```python
from build123d import *

# Parameters (mm, degrees)
ESTRUSIONE_ESTRUSIONE1_DEPTH                         = 25
SCHIZZO3_R                                           = 7
ESTRUSIONE_ESTRUSIONE2_DEPTH                         = 14.91
FORO_LAMATO_PER_VITE_M8_A_TESTA_CILINDRI_D           = 9
FORO_LAMATO_PER_VITE_M8_A_TESTA_CILINDRI_DEPTH       = 34.91
FORO_LAMATO_PER_VITE_M8_A_TESTA_CILINDRI_CBORE_D     = 15
FORO_LAMATO_PER_VITE_M8_A_TESTA_CILINDRI_CBORE_DEPTH = 8.6
TAGLIO_ESTRUSIONE3_DEPTH                             = 150
TAGLIO_ESTRUSIONE4_DEPTH                             = 30
TAGLIO_ESTRUSIONE5_START                             = -20
TAGLIO_ESTRUSIONE5_DEPTH                             = 20
TAGLIO_ESTRUSIONE6_DEPTH                             = 180
TAGLIO_ESTRUSIONE7_START                             = -5
TAGLIO_ESTRUSIONE7_DEPTH                             = 5
TAGLIO_ESTRUSIONE8_DEPTH                             = 2


with BuildPart() as part:
    # Schizzo2 → Estrusione-Estrusione1 (new body)
    with BuildSketch(Plane.XY):
        Polygon((0, 0), (-88, 0), (-88, -200), (-48, -200), (-48, -170), (-68, -170), (-68, -20), (0, -20), align=None)
    extrude(amount=ESTRUSIONE_ESTRUSIONE1_DEPTH)

    # Schizzo3 → Estrusione-Estrusione2 (add)
    with BuildSketch(Plane(origin=(0, 0, 0), x_dir=(1, 0, 0), z_dir=(0, 1, 0))):
        with Locations(Location((-41, -12.5, 0), (0, 0, 180))):
            Circle(SCHIZZO3_R)
        with Locations((-9, -12.5)):
            Circle(SCHIZZO3_R)
    extrude(amount=ESTRUSIONE_ESTRUSIONE2_DEPTH)

    # Foro lamato per Vite M8 a testa cilindrica-1
    with Locations(Plane(origin=(0, -20, 0), x_dir=(-1, 0, 0), z_dir=(0, -1, 0))):
        with Locations((9, -12.5), (41, -12.5)):
            CounterBoreHole(FORO_LAMATO_PER_VITE_M8_A_TESTA_CILINDRI_D / 2, FORO_LAMATO_PER_VITE_M8_A_TESTA_CILINDRI_CBORE_D / 2, FORO_LAMATO_PER_VITE_M8_A_TESTA_CILINDRI_CBORE_DEPTH, depth=FORO_LAMATO_PER_VITE_M8_A_TESTA_CILINDRI_DEPTH)

    # Schizzo10 → Taglio-Estrusione3 (cut)
    with BuildSketch(Plane(origin=(0, -170, 0), x_dir=(1, 0, 0), z_dir=(0, 1, 0))):
        with BuildLine():
            Line((-68, 0), (-72.387505004, 0))
            ThreePointArc((-72.387505004, 0), (-69.128726859, -5.876175573), (-68, -12.5))
            Line((-68, -12.5), (-68, 0))
        make_face()
        with BuildLine():
            Line((-68, -25), (-68, -12.5))
            ThreePointArc((-68, -12.5), (-69.128726859, -19.123824427), (-72.387505004, -25))
            Line((-72.387505004, -25), (-68, -25))
        make_face()
    extrude(amount=TAGLIO_ESTRUSIONE3_DEPTH, mode=Mode.SUBTRACT)

    # Schizzo11 → Taglio-Estrusione4 (cut)
    with BuildSketch(Plane(origin=(0, -170, 0), x_dir=(1, 0, 0), z_dir=(0, 1, 0))):
        with BuildLine():
            Line((-48, -25), (-48, 0))
            Line((-48, 0), (-71.125462969, 0))
            ThreePointArc((-71.125462969, 0), (-70.769833543, -0.494944237), (-70.428716609, -1))
            ThreePointArc((-70.428716609, -1), (-67, -12.5), (-70.428716609, -24))
            ThreePointArc((-70.428716609, -24), (-70.769833543, -24.505055763), (-71.125462969, -25))
            Line((-71.125462969, -25), (-48, -25))
        make_face()
    extrude(amount=-TAGLIO_ESTRUSIONE4_DEPTH, mode=Mode.SUBTRACT)

    # Schizzo12 → Taglio-Estrusione5 (cut)
    with BuildSketch(Plane.XZ.offset(200).offset(TAGLIO_ESTRUSIONE5_START)):
        with BuildLine():
            Line((-71.125462969, 25), (-88, 25))
            Line((-88, 25), (-88, 0))
            Line((-88, 0), (-71.125462969, 0))
            ThreePointArc((-71.125462969, 0), (-67, 12.5), (-71.125462969, 25))
        make_face()
    extrude(amount=TAGLIO_ESTRUSIONE5_DEPTH, mode=Mode.SUBTRACT)

    # Schizzo13 → Taglio-Estrusione6 (cut)
    with BuildSketch(Plane.XZ.offset(180)):
        Polygon((-88, 25), (-88, 12.5), (-84, 12.5), (-76.783121635, 25), align=None)
        Polygon((-84, 12.5), (-88, 12.5), (-88, 0), (-76.783121635, 0), align=None)
    extrude(amount=-TAGLIO_ESTRUSIONE6_DEPTH, mode=Mode.SUBTRACT)

    # Schizzo14 → Taglio-Estrusione7 (cut)
    with BuildSketch(Plane.XZ.offset(180).offset(TAGLIO_ESTRUSIONE7_START)):
        with BuildLine():
            Line((-76.783121635, 25), (-84, 12.5))
            Line((-84, 12.5), (-76.783121635, 0))
            Line((-76.783121635, 0), (-71.125462969, 0))
            ThreePointArc((-71.125462969, 0), (-67, 12.5), (-71.125462969, 25))
            Line((-71.125462969, 25), (-76.783121635, 25))
        make_face()
    extrude(amount=TAGLIO_ESTRUSIONE7_DEPTH, mode=Mode.SUBTRACT)

    # Schizzo15 → Taglio-Estrusione8 (cut)
    with BuildSketch(Plane(origin=(0, 0, 0), x_dir=(1, 0, 0), z_dir=(0, 1, 0))):
        Polygon((-76.783121635, -25), (-50, -25), (-50, 0), (-76.783121635, 0), (-84, -12.5), align=None)
    extrude(amount=-TAGLIO_ESTRUSIONE8_DEPTH, mode=Mode.SUBTRACT)


solid = part.part
```
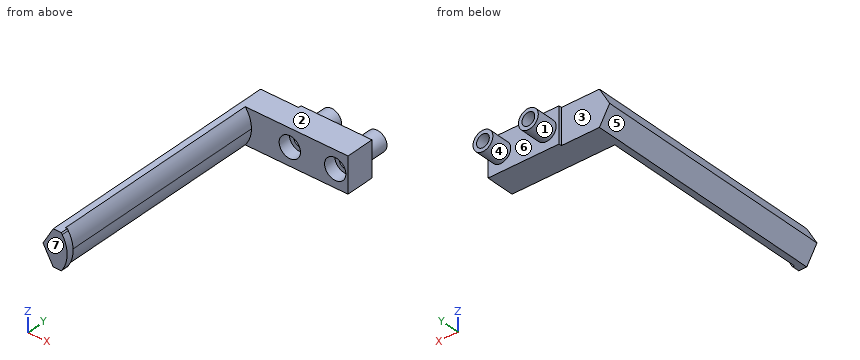
For this review, take the finished solid that the model builds, in its own axes (mm). Face numbers are marked on the shaded views. A direction names the side the tool comes from. Round coordinates to 2 decimals unless told otherwise and drop trailing zeros. Write each loop counter-clockwise with the first axis right and the second up, starting at its lowest first coordinate (ties: lowest second). Pieces come first, ordered by that corner, then holes. Notation, with made-up numbers: (3, 89.25) - (57, 89.25) arc R9 ccw to (57, 99.25) - close; hole circle Ø6 at (24.25, 83.5). An arc over 180 degrees is marked (long way). Put each result on its own line as item: value.
Q1. Insertion check: pin 1 Ø12.5 at (x, z) = (-52, 14) entering from -Y; pin 2 Ø14.5 at (x, z) = (-9, 12.5) entering from +Y; pin 3 Ø2.5 at (x, z) = (-69, 10.5) entering from +Y; pin 4 Ø1 at (y, z) = (-0.5, 14) entering from -X. Each pin has a flat end and moves straight along its axis. Give the tip position at first contact, or say it passes through.
Solved:
pin 1: stops at y = -20
pin 2: stops at y = 14.91
pin 3: stops at y = -2
pin 4: stops at x = -50
Q2. We need section C-C (x = -57). Give the boundary of the cut face in (y, z).
Solved:
outline: (-20, 0) - (-2, 0) - (-2, 25) - (-20, 25) - close
Q3. Mouldability with a two-part tool opening along X and no side actions: class the marked faces 4, 5, 6 and 7 as released by +X, released by -X, zero draft, split by the parting line, or undercut.
Solved:
face 4: undercut
face 5: released by -X
face 6: undercut
face 7: zero draft
Q4. Machinability: for the marked faces 1, 2 and 3, which of the approach directions +Z, -Z, +X, -X, +Y, -Y give a long, thin tool a straight path to every point of the face, cutting with its end or side? Answer none if there is none.
Solved:
face 1: +Y
face 2: +Z, +X, -X, +Y, -Y
face 3: +Z, -Z, -X, +Y
Q5. We need section B-B (y = 3). Give the boundary of the cut face in (x, z).
Solved:
outline: circle Ø14 at (-41, 12.5); circle Ø14 at (-9, 12.5); hole circle Ø9 at (-41, 12.5); hole circle Ø9 at (-9, 12.5)
Q6. We need section A-A (x = -41). Give the boundary of the cut face in (y, z).
Solved:
outline: (-20, 0) - (0, 0) - (0, 5.5) - (14.91, 5.5) - (14.91, 8) - (-11.4, 8) - (-11.4, 5) - (-20, 5) - close; (-20, 20) - (-11.4, 20) - (-11.4, 17) - (14.91, 17) - (14.91, 19.5) - (0, 19.5) - (0, 25) - (-20, 25) - close
Q7. We need section D-D (y = -103). Give the boundary of the cut face in (x, z).
Solved:
outline: (-84, 12.5) - (-76.78, 0) - (-72.39, 0) arc R20 ccw to (-72.39, 25) - (-76.78, 25) - close
Q8. Wall thickness on probe 1 along Z at (x, y) = (-41, -15); probe 2 along Z at (x, y) = (-41, 3); probe 3 along Y at (x, z) = (-14, 21.25): over which ranges is each line inside the solid? List them lowest first.
Solved:
probe 1: z = 0 to 5, 20 to 25
probe 2: z = 5.5 to 8, 17 to 19.5
probe 3: y = -20 to 0
